CAD build for the part. Positions are in the model's coordinates, mm. A direction names the side the tool comes from. Coordinates: 2 decimals unless noted, no trailing zeros. Order: outer loops, then holes, each group sorted by start corner. A loop starts at its lowest first (then second) coordinate and runs counter-clockwise, first axis right, second up. Notation, with made-up numbers: (-14, 27) - (-9, 27) arc R29 ccw to (-9, 48) - close; hole circle Ø7 at (79.5, 70). An arc over 180 degrees is marked (long way). Use one line per item in the form item = value.
```python
from build123d import *

# Parameters (mm, degrees)
SKETCH2_W           = 8
SKETCH2_H           = 19
SKETCH2_W_2         = 3
SKETCH2_H_2         = 3
BOSS_EXTRUDE1_DEPTH = 8
SKETCH2_3_W         = 3
SKETCH2_3_H         = 3
BOSS_EXTRUDE2_DEPTH = 3
SKETCH3_R           = 3.5
CUT_EXTRUDE1_DEPTH  = 1


with BuildPart() as part:
    # Sketch2 → Boss-Extrude1 (new body)
    with BuildSketch(Plane(origin=(0, 0, 0), x_dir=(1, 0, 0), z_dir=(0, 1, 0))):
        Rectangle(SKETCH2_W, SKETCH2_H)
        with Locations((0, 7)):
            Rectangle(SKETCH2_W_2, SKETCH2_H_2, mode=Mode.SUBTRACT)
        with Locations((0, 7)):
            Rectangle(SKETCH2_W_2, SKETCH2_H_2)
    extrude(amount=-BOSS_EXTRUDE1_DEPTH)

    # Sketch2_3 → Boss-Extrude2 (add)
    with BuildSketch(Plane(origin=(0, 0, 0), x_dir=(1, 0, 0), z_dir=(0, 1, 0))):
        with Locations((0, 7)):
            Rectangle(SKETCH2_3_W, SKETCH2_3_H)
    extrude(amount=BOSS_EXTRUDE2_DEPTH)

    # Sketch3 → Cut-Extrude1 (cut)
    with BuildSketch(Plane(origin=(0, 0, -9.5), x_dir=(-1, 0, 0), z_dir=(0, 0, -1))):
        with Locations((0, -4)):
            Circle(SKETCH3_R)
    extrude(amount=-CUT_EXTRUDE1_DEPTH, mode=Mode.SUBTRACT)


solid = part.part
```
Item 1: Drop flat-ended pins along their axis: pin 1 (2.5 mm diameter, centred on y = 1.5, z = -7, fed in from -X); pin 2 (0.9 mm diameter, centred on x = -0.5, y = 2, fed in from -Z); pin 3 (2.5 mm diameter, centred on y = 1.5, z = -6.5, fed in from +X). Give the stop position or say it passes through.
Derived:
pin_1 = -1.5
pin_2 = -8.5
pin_3 = 1.5
Item 2: Cut at D-D, the plane y = 1.75. Write the cut outline in (x, z), plus the area to 3 significant figures.
Derived:
outline = (-1.5, -8.5) - (1.5, -8.5) - (1.5, -5.5) - (-1.5, -5.5) - close
area = 9.00 mm²
Item 3: 3-axis set-ups, long thin cutter, end or side, ignore diameter. For faces 1 (the face through (0, 1, -5.5)), 2 (the face through (0, 1, -8.5)), 3 (the face through (-1.5, 1, -7)), 4 (the face through (0, -4, -8.5)): which of +Z, -Z, +X, -X, +Y, -Y reach the whole face in a straight line?
Derived:
face_1 = +Z, +X, -X, +Y
face_2 = -Z, +X, -X, +Y
face_3 = +Z, -Z, -X, +Y
face_4 = -Z
Item 4: Cut at C-C, the plane x = 0. Write the cut outline in (y, z).
Derived:
outline = (-8, -9.5) - (-7.5, -9.5) - (-7.5, -8.5) - (-0.5, -8.5) - (-0.5, -9.5) - (0, -9.5) - (0, -8.5) - (3, -8.5) - (3, -5.5) - (0, -5.5) - (0, 9.5) - (-8, 9.5) - close
Item 5: Cut at B-B, the plane z = -5.75. Write the cut outline in (x, y), plus the area to 3 significant figures.
Derived:
outline = (-4, -8) - (4, -8) - (4, 0) - (1.5, 0) - (1.5, 3) - (-1.5, 3) - (-1.5, 0) - (-4, 0) - close
area = 73.0 mm²
Item 6: Two-plate mould, pull along Y, no slides. Class faces 5 (the face through (0, 3, -7)), 6 (the face through (1.5, 1, -7)), 7 (the face through (0.759, -7.417, -9.007)): +Y half, -Y half, draft (parallel to the pull), parting line (faces both ways), or undercut.
Derived:
face_5 = +Y half
face_6 = draft
face_7 = undercut
Item 7: Cut at A-A, the plane y = -4. Write the cut outline in (x, z), plus the area to 3 significant figures.
Derived:
outline = (-4, -9.5) - (-3.5, -9.5) - (-3.5, -8.5) - (3.5, -8.5) - (3.5, -9.5) - (4, -9.5) - (4, 9.5) - (-4, 9.5) - close
area = 145 mm²
Item 8: Drill centre lines: line 1 (Y direction, x = 0, z = -8.7); line 2 (Y direction, x = 3, z = 4.75); line 3 (Z direction, x = 0, y = -2.5). Where is each one in solid material? Low to high. Write a range as [from, to].
Derived:
line_1 = [-8, -7.5], [-0.5, 0]
line_2 = [-8, 0]
line_3 = [-8.5, 9.5]
